Source: three-view drawing plus pictorial views. Frame: mm from the lowest corner of the part. Give positions to 0.01 mm unless a question says otherwise; leave off trailing zeros. Loops run counter-clockwise (first coordinate to the right, second up) from the corner with the lowest first, then second, coordinate; pieces in that order, holes last. Notation, with made-up numbers: (68, -23.75) - (106, -23.75) arc R22 cw to (106, 2.25) - close; hole circle Ø4 at (-25, 13.5). An arc over 180 degrees is marked (long way). One line per item, written item: value.
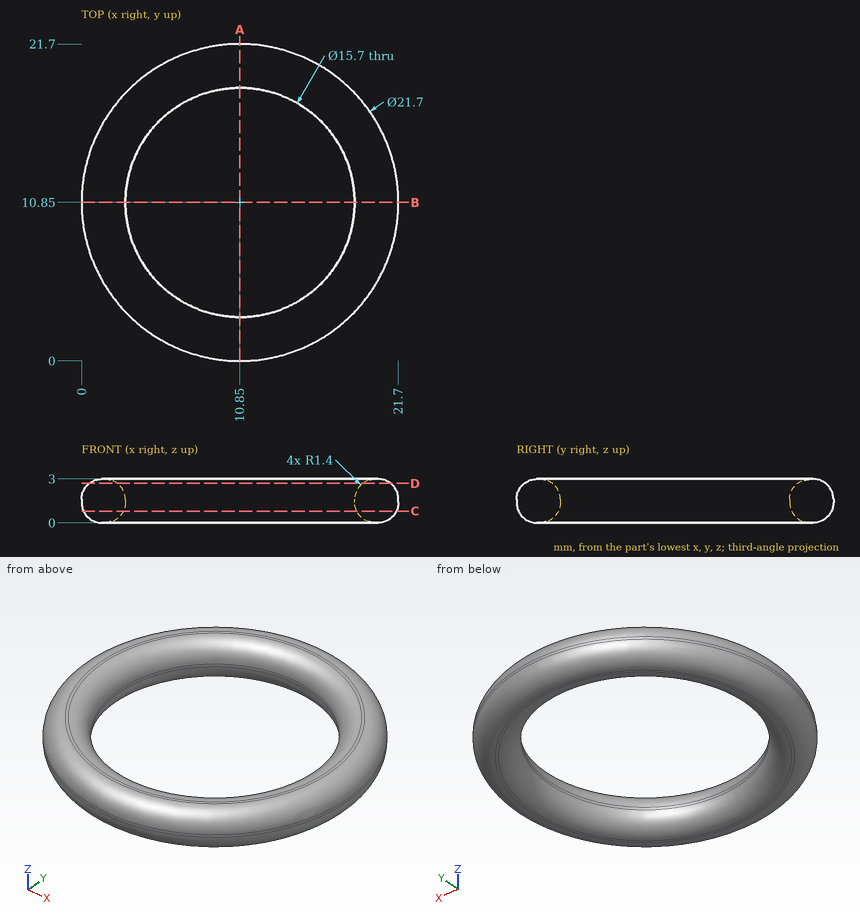
Item 1: Section D-D, the plane z = 2.7. Output: boundary loops of the cut face in (x, y), and give its area (3 significant figures).
Verdict:
outline: circle Ø20.63 at (10.85, 10.85); hole circle Ø16.77 at (10.85, 10.85)
area: 114 mm^2
Item 2: Section A-A, the plane x = 10.85. Output: boundary loops of the cut face in (y, z), and give its area (3 significant figures).
Verdict:
outline: (0, 1.4) arc R1.4 ccw to (1.4, 0) - (1.6, 0) arc R1.4 ccw to (3, 1.4) - (3, 1.6) arc R1.4 ccw to (1.6, 3) - (1.4, 3) arc R1.4 ccw to (0, 1.6) - close; (18.7, 1.4) arc R1.4 ccw to (20.1, 0) - (20.3, 0) arc R1.4 ccw to (21.7, 1.4) - (21.7, 1.6) arc R1.4 ccw to (20.3, 3) - (20.1, 3) arc R1.4 ccw to (18.7, 1.6) - close
area: 14.6 mm^2
Item 3: Material intervals for L1, parallel to Y at x = 10.85, z = 1.55; L2, parallel to X at y = 5.5, z = 1.85; L3, parallel to Y at x = 5.5, z = 2.1, sorted ascending.
Verdict:
L1: y = 0 to 3, 18.7 to 21.7
L2: x = 1.44 to 5.07, 16.63 to 20.26
L3: y = 1.52 to 4.98, 16.72 to 20.18
Item 4: Section C-C, the plane z = 0.8. Output: boundary loops of the cut face in (x, y).
Verdict:
outline: circle Ø21.43 at (10.85, 10.85); hole circle Ø15.97 at (10.85, 10.85)
Item 5: Pin query (flat end, axial travel): P1, Ø1, axis at x = 8, z = 0.5, coming from the +Y side; P2, Ø2, axis at x = 4, y = 19, coming from the -Z side. Return the tip coordinate at first contact, or that it passes through.
Verdict:
P1: stops at y = 21.3
P2: stops at z = 0.01
